```python
from build123d import *

# Parameters (mm, degrees)
F0_W     = 101.6
F0_H     = 558.8
F0_W_2   = 18.542
F0_H_2   = 101.6
F0_W_3   = 152.4
F0_W_4   = 381
F0_H_3   = 381
F0_R     = 19.05
F1_DEPTH = 25.4


with BuildPart() as f1:
    # F0 (on Top) → F1 (new body)
    with BuildSketch(Plane.XY):
        Polygon((381, -762), (381, 762), (190.5, 762), (-190.5, 762), (-381, 762), (-381, -762), align=None)
        with Locations((-228.6, -381)):
            Rectangle(F0_W, F0_H, mode=Mode.SUBTRACT)
        with Locations((-130.175, -50.8)):
            Rectangle(F0_W_2, F0_H_2, mode=Mode.SUBTRACT)
        with Locations((0, -381)):
            Rectangle(F0_W_3, F0_H, mode=Mode.SUBTRACT)
        with Locations((228.6, -381)):
            Rectangle(F0_W, F0_H, mode=Mode.SUBTRACT)
        with Locations((130.175, -50.8)):
            Rectangle(F0_W_2, F0_H_2, mode=Mode.SUBTRACT)
        with Locations((0, 952.5)):
            Rectangle(F0_W_4, F0_H_3)
        with Locations((0, 952.5)):
            Circle(F0_R, mode=Mode.SUBTRACT)
    extrude(amount=F1_DEPTH)


solid = f1.part
```
Build history of the part. All positions in model axes, mm. Give positions to 0.01 mm unless a question says otherwise; leave off trailing zeros. Loops run counter-clockwise (first coordinate to the right, second up) from the corner with the lowest first, then second, coordinate; pieces in that order, holes last.
1) Probe line 1 along X through (y, z) = (-492, 10.75); line 2 along Y through (x, z) = (0, 14.25); line 3 along Y through (x, z) = (-124, 22.25). List the from-to ranges inside material, lowest first.
Values follow:
line 1: x = -381 to -279.4, -177.8 to -76.2, 76.2 to 177.8, 279.4 to 381
line 2: y = -762 to -660.4, -101.6 to 933.45, 971.55 to 1143
line 3: y = -762 to -101.6, 0 to 1143
2) Band-saw the part on C-C on z = 10.25. State how many separate pieces and enclosed holes the cut face has, then the cut area to 3 significant figures.
Values follow:
separate pieces: 1
enclosed holes: 6
area: 1,100,000 mm2
3) Drop flat-ended pins along their axis: P1, Ø6, axis at x = -56, y = 383, coming from the -Z side; P2, Ø4, axis at x = 216.5, z = 7, coming from the +Y side. Give the stop position or say it passes through.
Values follow:
P1: stops at z = 0
P2: stops at y = 762
4) Band-saw the part on A-A on y = 952.5. List the corners of the cut face in (x, z), then the cut area to 3 significant figures.
Values follow:
outline: (-190.5, 0) - (-19.05, 0) - (-19.05, 25.4) - (-190.5, 25.4) - close; (19.05, 0) - (190.5, 0) - (190.5, 25.4) - (19.05, 25.4) - close
area: 8,710 mm2
5) Two-plate mould, pull along X, no slides. Class faces 1 (the face through (-2.48, 971.388, 12.522)), 2 (the face through (-5, 204, 25.4)): released by +X, released by -X, zero draft, split by the parting line, or undercut.
Values follow:
face 1: undercut
face 2: zero draft
6) Band-saw the part on B-B on x = 0. List the corners of the cut face in (y, z), then the cut area to 3 significant figures.
Values follow:
outline: (-762, 0) - (-660.4, 0) - (-660.4, 25.4) - (-762, 25.4) - close; (-101.6, 0) - (933.45, 0) - (933.45, 25.4) - (-101.6, 25.4) - close; (971.55, 0) - (1143, 0) - (1143, 25.4) - (971.55, 25.4) - close
area: 33,200 mm2
7) Band-saw the part on D-D on y = -152.5. List the corners of the cut face in (x, z), then the cut area to 3 significant figures.
Values follow:
outline: (-381, 0) - (-279.4, 0) - (-279.4, 25.4) - (-381, 25.4) - close; (-177.8, 0) - (-76.2, 0) - (-76.2, 25.4) - (-177.8, 25.4) - close; (76.2, 0) - (177.8, 0) - (177.8, 25.4) - (76.2, 25.4) - close; (279.4, 0) - (381, 0) - (381, 25.4) - (279.4, 25.4) - close
area: 10,300 mm2
